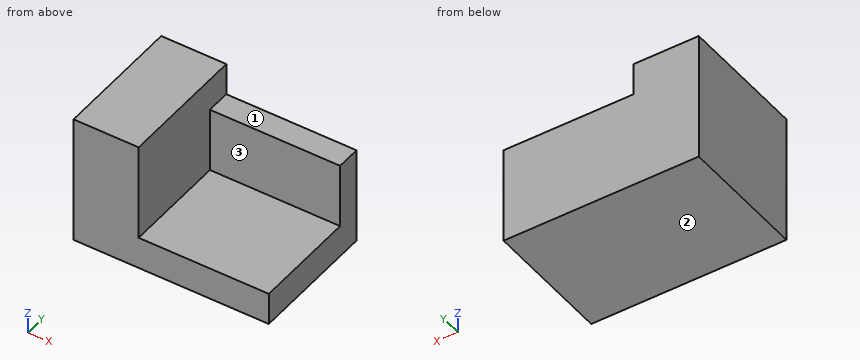
```python
from build123d import *

# Parameters (mm, degrees)
F1_DEPTH = 25.4
F2_W     = 4.7399289906
F2_H     = 12.7
F3_DEPTH = 25.4


with BuildPart() as f1:
    # F0 (on Front) → F1 (new body)
    with BuildSketch(Plane.XZ):
        Polygon((0, 25.4), (0, 0), (38.1, 0), (38.1, 6.35), (12.7, 6.35), (12.7, 25.4), align=None)
    extrude(amount=F1_DEPTH)

    # F2 (on face) → F3 (join)
    with BuildSketch(Plane.YZ.offset(12.7)):
        with Locations((-2.3699644953, 12.7)):
            Rectangle(F2_W, F2_H)
    extrude(amount=F3_DEPTH)


solid = f1.part
```
CAD build for the part. Positions are in the model's coordinates, mm. Face numbers are marked on the shaded views. A direction names the side the tool comes from. Round coordinates to 2 decimals unless told otherwise and drop trailing zeros. Write each loop counter-clockwise with the first axis right and the second up, starting at its lowest first coordinate (ties: lowest second). Pieces come first, ordered by that corner, then holes.
Item 1: Band-saw the part on A-A on x = 19. Write the cut outline in (y, z).
Filled in:
outline: (-25.4, 0) - (0, 0) - (0, 19.05) - (-4.74, 19.05) - (-4.74, 6.35) - (-25.4, 6.35) - close
Item 2: Band-saw the part on B-B on y = -18.75. Write the cut outline in (x, z).
Filled in:
outline: (0, 0) - (38.1, 0) - (38.1, 6.35) - (12.7, 6.35) - (12.7, 25.4) - (0, 25.4) - close
Item 3: Drop flat-ended pins along their axis: pin 1 Ø6.5 at (x, z) = (29.5, 14) entering from -Y; pin 2 Ø2 at (y, z) = (-9, 12.5) entering from +X; pin 3 Ø2.5 at (x, y) = (23, -2) entering from +Z. Give the stop position or say it passes through.
Filled in:
pin 1: stops at y = -4.74
pin 2: stops at x = 12.7
pin 3: stops at z = 19.05
Item 4: Drill centre lines: L1, parallel to Y at x = 34, z = 12.5; L2, parallel to Z at x = 22.5, y = -16.5; L3, parallel to X at y = -8, z = 20. Where is each one in solid material? Low to high.
Filled in:
L1: y = -4.74 to 0
L2: z = 0 to 6.35
L3: x = 0 to 12.7
Item 5: Band-saw the part on C-C on z = 21. Write the cut outline in (x, y), then the cut area to 3 significant figures.
Filled in:
outline: (0, -25.4) - (12.7, -25.4) - (12.7, 0) - (0, 0) - close
area: 323 mm2
Item 6: Tool access for the marked faces 1, 2 and 3: list every direction of +Z, -Z, +X, -X, +Y, -Y with a clear straight run to the whole face (end or side of a thin tool).
Filled in:
face 1: +Z, +X, +Y, -Y
face 2: -Z, +X, -X, +Y, -Y
face 3: +Z, +X, -Y
